Answer from the drawing. Dimensions are ordinates in mm from the lowest x, y and z of the part. A direction names the side the tool comes from. Give positions to 0.01 mm unless a question says otherwise; leave off trailing zeros. Order: outer loops, then holes, each group sorted by start corner. A loop starts at its lowest first (then second) coordinate and runs counter-clockwise, first axis right, second up. Notation, with made-up numbers: M 63,-30 L 78,-30 A19 cw 78,0 Z; hole C 21.5,-36 d2. An arc over 180 degrees is marked long. One line per item, written item: value.
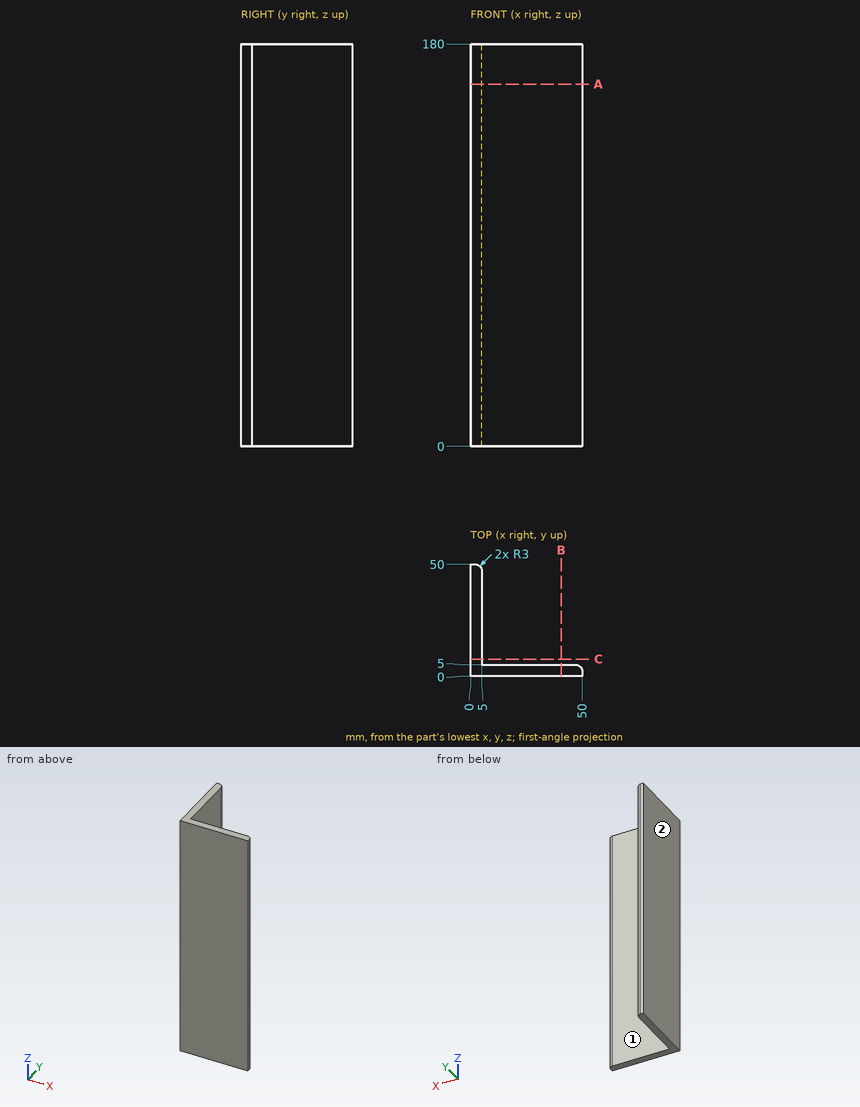
(1) Which of the six approach directions +Z, -Z, +X, -X, +Y, -Y give full straight-line access (tool end or side, diameter ignored) to the marked faces 1 and 2?
Findings:
face 1: +Z, -Z, +X, +Y
face 2: +Z, -Z, -X, +Y, -Y
(2) Given P1, Ø1, axis at x = 10.5, z = 48.5, coming from the +Y side; P2, Ø12.5, axis at y = 22, z = 74.5, coming from the +X side, each flat-ended and moving along its own axis, determine where each tip first touches the part or whether it passes through.
Findings:
P1: stops at y = 5
P2: stops at x = 5
(3) Section B-B, the plane x = 40.5 is taken. Give the vertices of the cut face in (y, z).
Findings:
outline: M 0,0 L 5,0 L 5,180 L 0,180 Z
(4) Section A-A, the plane z = 162 is taken. Give the vertices of the cut face in (x, y), then the cut area to 3 significant figures.
Findings:
outline: M 0,0 L 50,0 L 50,2 A3 ccw 47,5 L 5,5 L 5,47 A3 ccw 2,50 L 0,50 Z
area: 471 mm^2
(5) Find the intervals of material crossed by probe 1 along X at (y, z) = (10.5, 14); probe 2 along X at (y, z) = (3.5, 97), in increasing order. Write a range as from..to.
Findings:
probe 1: x = 0..5
probe 2: x = 0..49.6
